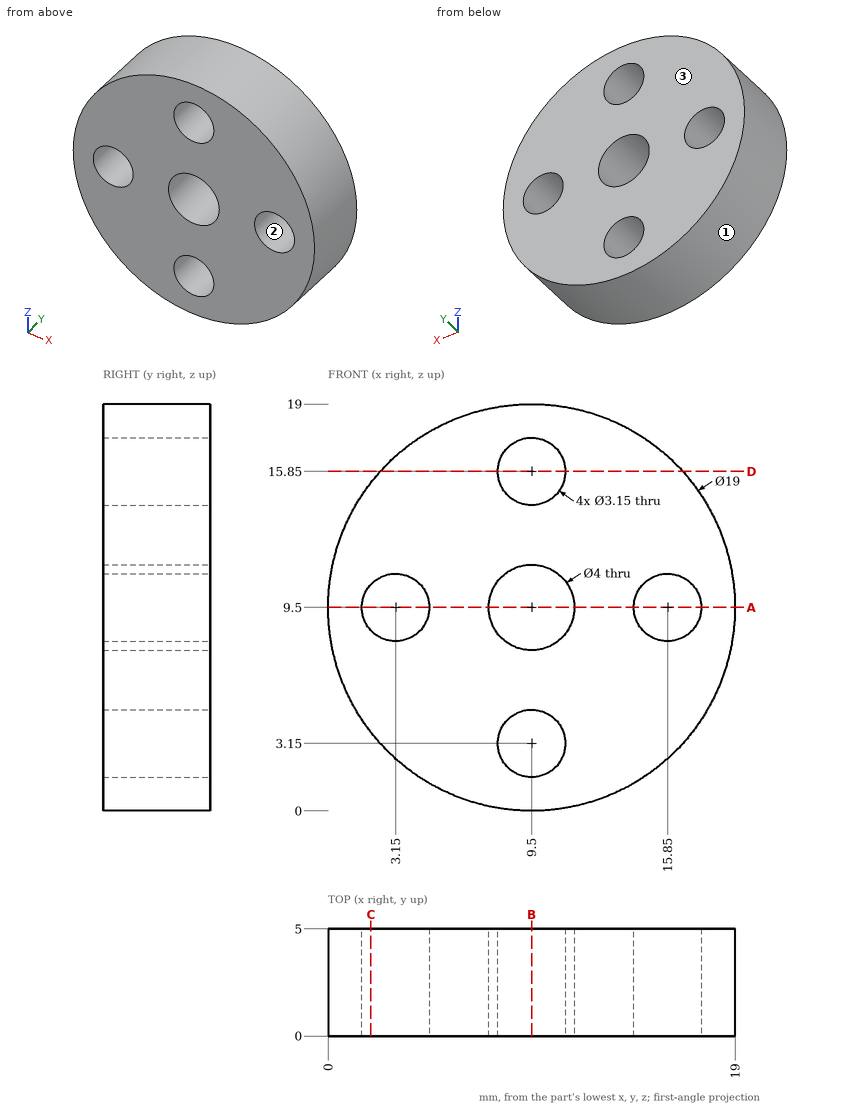
For this review, use the dimensioned drawing (mm, ordinates from the lowest corner) and the shaded views. Give positions to 0.01 mm unless a question says otherwise; leave off trailing zeros. Write each loop counter-clockwise with the first axis right and the second up, starting at its lowest first coordinate (ties: lowest second). Pieces come first, ordered by that corner, then holes. Notation, with made-up numbers: M 73,32 L 97,32 A26 ccw 97,64 Z; hole C 87,65.25 d3. An arc over 180 degrees is marked long. Write item = value, one per line. Start each with the question number.
Q1. Mouldability with a two-part tool opening along Z and no side actions: class the marked faces 1, 2 and 3 as released by +Z, released by -Z, zero draft, split by the parting line, or undercut.
Q2. We need section D-D (z = 15.85). State the section outline as (x, y) points (3 decimals).
Q3. For line 1 (Z direction, x = 9.5, y = 4.15) (3 decimals); line 2 (Z direction, x = 4.25, y = 3.4), list the stretches that pass through material, from the lowest coordinate up.
Q4. We need section C-C (x = 2). State the section outline as (y, z) points, plus the area to 3 significant figures.
Q5. We need section A-A (z = 9.5). State the section outline as (x, y) points (3 decimals), plus the area to 3 significant figures.
Q6. Clearance check with a flat-ended pin moving along its axis: pin 1 (3 mm diameter, centred on y = 1.5, z = 2.5, fed in from +X). State where the tip first meets the part, or that it passes through.
Q7. We need section B-B (x = 9.5). State the section outline as (y, z) points (3 decimals).
Result set:
q1.face_1 = split by the parting line
q1.face_2 = undercut
q1.face_3 = zero draft
q2.outline = M 2.434,0 L 7.925,0 L 7.925,5 L 2.434,5 Z; M 11.075,0 L 16.566,0 L 16.566,5 L 11.075,5 Z
q3.line_1 = 0 to 1.575, 4.725 to 7.5, 11.5 to 14.275, 17.425 to 19
q3.line_2 = 1.58 to 8.37, 10.63 to 17.42
q4.outline = M 0,3.67 L 5,3.67 L 5,8.42 L 0,8.42 Z; M 0,10.58 L 5,10.58 L 5,15.33 L 0,15.33 Z
q4.area = 47.5 mm2
q5.outline = M 0,0 L 1.575,0 L 1.575,5 L 0,5 Z; M 4.725,0 L 7.5,0 L 7.5,5 L 4.725,5 Z; M 11.5,0 L 14.275,0 L 14.275,5 L 11.5,5 Z; M 17.425,0 L 19,0 L 19,5 L 17.425,5 Z
q5.area = 43.5 mm2
q6.pin_1 = 17.25
q7.outline = M 0,0 L 5,0 L 5,1.575 L 0,1.575 Z; M 0,4.725 L 5,4.725 L 5,7.5 L 0,7.5 Z; M 0,11.5 L 5,11.5 L 5,14.275 L 0,14.275 Z; M 0,17.425 L 5,17.425 L 5,19 L 0,19 Z
